from build123d import *

# Parameters (mm, degrees)
F1_W     = 43.6626
F1_H     = 3.175
F2_DEPTH = 103.1875
F3_R     = 1.9812
F4_DEPTH = 107.95


# Not quite as in the source:
# - a variable given as a bare number and used for a length is read in inches; the dataset says mm whatever the document's units were


with BuildPart() as f2:
    # F1 (on Right) → F2 (new body, symmetric)
    with BuildSketch(Plane.YZ):
        Rectangle(F1_W, F1_H)
    extrude(amount=F2_DEPTH, both=True)

    # F3 (on Right) → F4 (join, symmetric)
    with BuildSketch(Plane.YZ):
        Circle(F3_R)
    extrude(amount=F4_DEPTH, both=True)


solid = f2.part
Verification items for the finished model (mm, model axes). A direction names the side the tool comes from. Round coordinates to 2 decimals unless told otherwise and drop trailing zeros. Loops run counter-clockwise (first coordinate to the right, second up) from the corner with the lowest first, then second, coordinate; pieces in that order, holes last. Notation, with made-up numbers: (58.25, 13) - (91.25, 13) arc R26 ccw to (91.25, 49) - close; hole circle Ø4 at (47.25, 27.25). An arc over 180 degrees is marked (long way). Answer in a Markdown table with one row per item. Add a question column.
Q1. Section check B-B on x = 49. Enter the section's corners in (y, z).
Q2. Section check C-C on y = 13. Enter the section's corners in (x, z).
Q3. Material ranges on line 1 (Z direction, x = 48, y = -10.5); line 2 (X direction, y = -17, z = -0.9); line 3 (Z direction, x = -47, y = 1), recorded low to high.
Q4. Gauge pin test, flat ends, axial feed: pin 1 (6 mm diameter, centred on x = -38.5, y = 13.5, fed in from -Z); pin 2 (10.5 mm diameter, centred on x = 23, y = -12, fed in from +Z); pin 3 (1 mm diameter, centred on y = -11.5, z = 0, fed in from -X). Record the tip position at first contact, or that the pin passes through.
Q5. Section check A-A on z = 0. Enter the section's corners in (x, y).
Q6. Tool access check on faces 1 (the face through (1, 11, -1.588)), 2 (the face through (1, -12, -1.588)), 3 (the face through (1, 11, 1.588)). Record the directions out of +Z, -Z, +X, -X, +Y, -Y that give a thin tool (end or side, any length) a straight path to the whole face; none if there is none.
Found:
| question | item | result |
|---|---|---|
| 1 | outline | (-21.83, -1.59) - (-1.19, -1.59) arc R1.98 ccw to (1.19, -1.59) - (21.83, -1.59) - (21.83, 1.59) - (1.19, 1.59) arc R1.98 ccw to (-1.19, 1.59) - (-21.83, 1.59) - close |
| 2 | outline | (-103.19, -1.59) - (103.19, -1.59) - (103.19, 1.59) - (-103.19, 1.59) - close |
| 3 | line 1 | z = -1.59 to 1.59 |
| 3 | line 2 | x = -103.19 to 103.19 |
| 3 | line 3 | z = -1.71 to 1.71 |
| 4 | pin 1 | stops at z = -1.59 |
| 4 | pin 2 | stops at z = 1.59 |
| 4 | pin 3 | stops at x = -103.19 |
| 5 | outline | (-107.95, -1.98) - (-103.19, -1.98) - (-103.19, -21.83) - (103.19, -21.83) - (103.19, -1.98) - (107.95, -1.98) - (107.95, 1.98) - (103.19, 1.98) - (103.19, 21.83) - (-103.19, 21.83) - (-103.19, 1.98) - (-107.95, 1.98) - close |
| 6 | face 1 | -Z, +X, -X, +Y |
| 6 | face 2 | -Z, +X, -X, -Y |
| 6 | face 3 | +Z, +X, -X, +Y |
